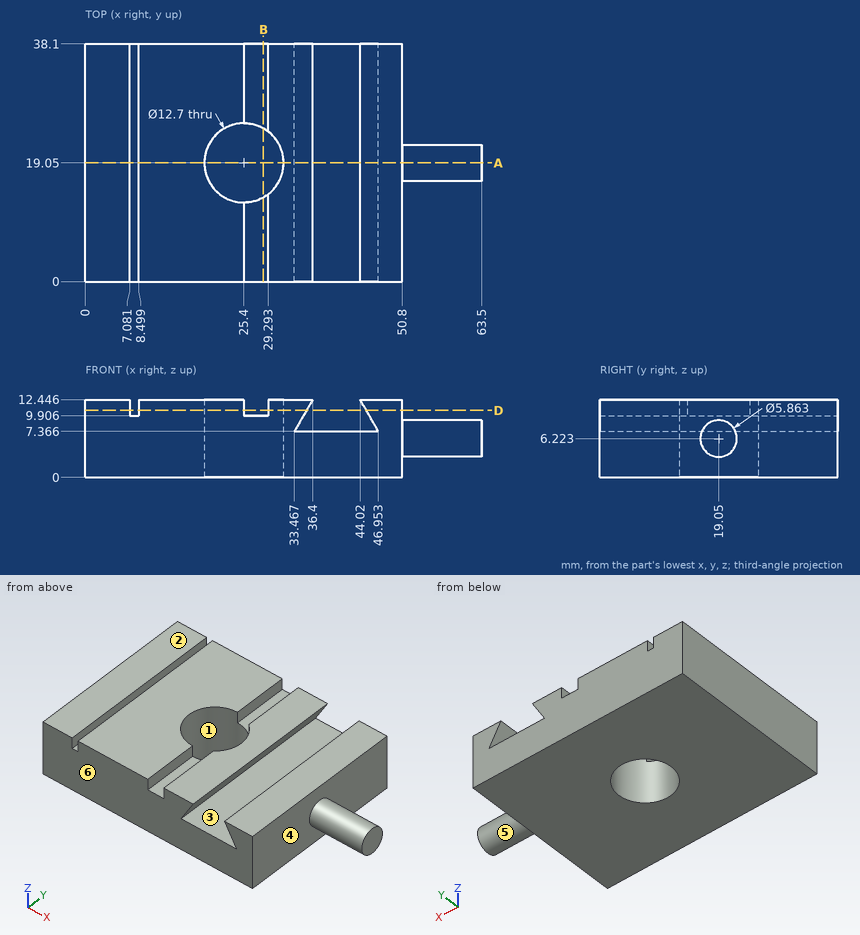
Check sheet for the drawn part. Datum: minimum x, y, z corner. Units: mm. A direction names the side the tool comes from. Coordinates: 2 decimals unless noted, no trailing zeros. Loops run counter-clockwise (first coordinate to the right, second up) from the corner with the lowest first, then second, coordinate; pieces in that order, holes last. Notation, with made-up numbers: (55.25, 39) -> (101.25, 39) arc R21 cw to (101.25, 62) -> close; hole circle Ø8 at (46, 20). An arc over 180 degrees is marked (long way). Answer in a Markdown table with one row per item.
1. Access from +Z, -Z, +X, -X, +Y, -Y to the whole of each face (thin tool, end or side, straight path). Record for the marked faces 5 and 6.
Check values:
| item | result |
|---|---|
| face 5 | +X |
| face 6 | +Z, -Z, +X, -X, -Y |
2. Sectioned sample at B-B, the plane x = 28.5. Record the boundary of the cut face in (y, z), then the cut area to 3 significant figures.
Check values:
| item | result |
|---|---|
| outline | (0, 0) -> (13.51, 0) -> (13.51, 9.91) -> (0, 9.91) -> close; (24.59, 0) -> (38.1, 0) -> (38.1, 9.91) -> (24.59, 9.91) -> close |
| area | 268 mm2 |
3. Material ranges on line 1 along Y through (x, z) = (25.4, 9.5); line 2 along X through (y, z) = (19.05, 4.75); line 3 along X through (y, z) = (19.05, 7.75), recorded low to high. Write a range as [from, to].
Check values:
| item | result |
|---|---|
| line 1 | y = [0, 12.7], [25.4, 38.1] |
| line 2 | x = [0, 19.05], [31.75, 63.5] |
| line 3 | x = [0, 19.05], [31.75, 33.69], [46.73, 63.5] |
4. Release check for a two-part mould opening along X. For the marked faces 1, 2, 3 and 4 record: released by +X, released by -X, zero draft, split by the parting line, or undercut.
Check values:
| item | result |
|---|---|
| face 1 | undercut |
| face 2 | zero draft |
| face 3 | undercut |
| face 4 | released by +X |
5. Sectioned sample at A-A, the plane y = 19.05. Record the boundary of the cut face in (x, z).
Check values:
| item | result |
|---|---|
| outline | (0, 0) -> (19.05, 0) -> (19.05, 12.45) -> (8.5, 12.45) -> (8.5, 9.91) -> (7.08, 9.91) -> (7.08, 12.45) -> (0, 12.45) -> close; (31.75, 0) -> (50.8, 0) -> (50.8, 3.29) -> (63.5, 3.29) -> (63.5, 9.15) -> (50.8, 9.15) -> (50.8, 12.45) -> (44.02, 12.45) -> (46.95, 7.37) -> (33.47, 7.37) -> (36.4, 12.45) -> (31.75, 12.45) -> close |
6. Go/stop test with flat-tipped pins: pin 1 (0.8 mm diameter, centred on y = 31, z = 11.5, fed in from +X); pin 2 (1.9 mm diameter, centred on x = 26.5, y = 28.5, fed in from +Z). Record where each tip stops, or that it passes through.
Check values:
| item | result |
|---|---|
| pin 1 | stops at x = 50.8 |
| pin 2 | stops at z = 9.91 |
7. Sectioned sample at D-D, the plane z = 10.75. Record the boundary of the cut face in (x, y).
Check values:
| item | result |
|---|---|
| outline | (0, 0) -> (7.08, 0) -> (7.08, 38.1) -> (0, 38.1) -> close; (8.5, 0) -> (25.4, 0) -> (25.4, 12.7) arc R6.35 cw to (25.4, 25.4) -> (25.4, 38.1) -> (8.5, 38.1) -> close; (29.29, 0) -> (35.42, 0) -> (35.42, 38.1) -> (29.29, 38.1) -> (29.29, 24.07) arc R6.35 cw to (29.29, 14.03) -> close; (45, 0) -> (50.8, 0) -> (50.8, 38.1) -> (45, 38.1) -> close |
